```python
from build123d import *

# Parameters (mm, degrees)
EXTRUDE_1_REACH          = 90.826
EXTRUDE_1_END_RADIUS     = 27
SKETCH_2_R               = 13
SKETCH_4_R               = 9
CUT_EXTRUDE_2_DEPTH      = 89.825671965
SKETCH_5_R               = 10
CUT_EXTRUDE_3_DEPTH      = 0.5
EXTRUDE_1_2_REACH        = 90.826
CUT_EXTRUDE_4_DEPTH      = 82.737384446
CUT_EXTRUDE_4_DEPTH_BACK = 82.737384446
SKETCH_6_W               = 70
SKETCH_6_H               = 5


with BuildPart() as part:
    # 草图1 → 旋转1 (revolve)
    with BuildSketch(Plane.XY, mode=Mode.PRIVATE) as revolve_1_sk:
        with BuildLine():
            Line((0, 53), (25, 53))
            ThreePointArc((25, 53), (28.535533906, 54.464466094), (30, 58))
            Line((30, 58), (30, 59))
            Line((30, 59), (40, 59))
            Line((40, 59), (40, 53))
            Line((40, 53), (37, 53))
            Line((37, 53), (37, 51))
            Line((37, 51), (40, 51))
            Line((40, 51), (40, 48))
            Line((40, 48), (37, 48))
            Line((37, 48), (37, 46))
            Line((37, 46), (40, 46))
            Line((40, 46), (40, 44))
            Line((40, 44), (37, 44))
            Line((37, 44), (37, 41))
            Line((37, 41), (40, 41))
            Line((40, 41), (40, 0))
            Line((40, 0), (27, 0))
            Line((27, 0), (27, 41.5))
            ThreePointArc((27, 41.5), (25.535533906, 45.035533906), (22, 46.5))
            Line((22, 46.5), (0, 46.5))
            Line((0, 46.5), (0, 53))
        make_face()
    revolve(revolve_1_sk.sketch.rotate(Axis((0, -5, 0), (0, 1, 0)), 90), axis=Axis((0, -5, 0), (0, 1, 0)))

    # Extrude 1: up to this cylinder (the profile starts inside it)
    extrude_1_end = Plane(origin=(0, 25, 0), z_dir=(0, -1, 0)) * Cylinder(EXTRUDE_1_END_RADIUS, 236.652, mode=Mode.PRIVATE)
    # 草图2 → Extrude 1 (add, up to the surface)
    with BuildSketch(Plane.XY.offset(13), mode=Mode.PRIVATE) as extrude_1_sk1:
        with Locations(Location((0, 25, 0), (0, 0, 180))):
            Circle(SKETCH_2_R)
    extrude_1_tool1 = extrude(extrude_1_sk1.sketch, amount=EXTRUDE_1_REACH, mode=Mode.PRIVATE) & extrude_1_end
    extrude_1 = extrude_1_tool1.solids().sort_by_distance((0, 25, 13))[0]
    add(extrude_1)

    # 草图4 → 切除-拉伸2 (cut, through all)
    with BuildSketch(Plane.XY.offset(13)):
        with Locations(Location((0, 25, 0), (0, 0, 270))):
            Circle(SKETCH_4_R)
    cut_extrude_2 = extrude(amount=CUT_EXTRUDE_2_DEPTH, mode=Mode.SUBTRACT)

    # 草图5 → 切除-拉伸3 (cut)
    with BuildSketch(Plane.XY.offset(38)):
        with Locations((0, 25)):
            Circle(SKETCH_5_R)
    cut_extrude_3 = extrude(amount=CUT_EXTRUDE_3_DEPTH, mode=Mode.SUBTRACT)

    # 草图7 → Extrude 1 2 (add, up to next)
    with BuildSketch(Plane(origin=(0, 0, 13), x_dir=(-1, 0, 0), z_dir=(0, 0, -1)), mode=Mode.PRIVATE) as extrude_1_2_sk1:
        with BuildLine():
            Line((-13, 25), (-13, 46.5))
            Line((-13, 46.5), (13, 46.5))
            Line((13, 46.5), (13, 25))
            ThreePointArc((13, 25), (0, 38), (-13, 25))
        make_face()
    extrude_1_2_tool1 = extrude(extrude_1_2_sk1.sketch, amount=-EXTRUDE_1_2_REACH, mode=Mode.PRIVATE) - part.part
    extrude_1_2 = extrude_1_2_tool1.solids().sort_by_distance((0, 40.482231, 13))[0]
    add(extrude_1_2)

    # 镜向1: Extrude 1, 切除-拉伸2, 切除-拉伸3, Extrude 1 2 across plane
    add(extrude_1.mirror(Plane.XY))
    add(cut_extrude_2.mirror(Plane.XY), mode=Mode.SUBTRACT)
    add(cut_extrude_3.mirror(Plane.XY), mode=Mode.SUBTRACT)
    add(extrude_1_2.mirror(Plane.XY))

    # 草图6 → 切除-拉伸4 (cut, two sides: drawn at the far end of the back side and taken through both)
    with BuildSketch(Plane.XY.offset(-CUT_EXTRUDE_4_DEPTH_BACK)):
        with Locations((0, 2.5)):
            Rectangle(SKETCH_6_W, SKETCH_6_H)
    extrude(amount=CUT_EXTRUDE_4_DEPTH + CUT_EXTRUDE_4_DEPTH_BACK, mode=Mode.SUBTRACT)


solid = part.part
```
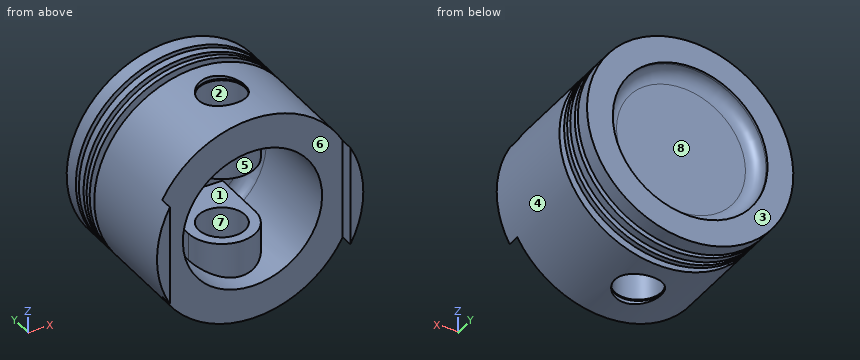
CAD build for the part. Positions are in the model's coordinates, mm. Face numbers are marked on the shaded views. A direction names the side the tool comes from. Round coordinates to 2 decimals unless told otherwise and drop trailing zeros. Order: outer loops, then holes, each group sorted by start corner. A loop starts at its lowest first (then second) coordinate and runs counter-clockwise, first axis right, second up.
Item 1: Mould opens along X. For the marked faces 1, 2, 3 and 4 say: pulls with the +X half, pulls with the -X half, needs draft (parallel to the pull), parting line crosses it, or undercut.
Item 2: Tool access for the marked faces 5, 6, 7 and 8: list every direction of +Z, -Z, +X, -X, +Y, -Y with a clear straight run to the whole face (end or side of a thin tool).
Item 3: Saw through at C-C on y = 8.5. Write the cut outline in (x, z), then the cut area to 3 significant figures.
Item 4: Saw through at B-B on x = 0. State how many separate pieces and enclosed holes the cut face has, then the cut area to 3 significant figures.
Item 5: Probe line 1 along Y through (x, z) = (0, 39); line 2 along Y through (x, z) = (-19, 32.5); line 3 along X through (y, z) = (25, 18). List the from-to ranges inside material, lowest first.
Item 6: Pin check, flat tips, straight feed: pin 1 (8.5 mm diameter, centred on y = 32, z = -17.5, fed in from +X); pin 2 (11 mm diameter, centred on x = 0, y = 25, fed in from -Z); pin 3 (4 mm diameter, centred on x = -6, y = 30, fed in from -Z); pin 4 (21 mm diameter, centred on x = 1, y = 26, fed in from -Z). Stop position of each tip, or through.
Reported:
1. face 1: undercut
1. face 2: undercut
1. face 3: needs draft
1. face 4: parting line crosses it
2. face 5: -Y
2. face 6: +Z, -Z, -Y
2. face 7: +Z, -Z
2. face 8: +Y
3. outline: circle Ø80 at (0, 0); hole circle Ø54 at (0, 0)
3. area: 2,740 mm2
4. separate pieces: 3
4. enclosed holes: 0
4. area: 1,680 mm2
5. line 1: y = 5 to 16, 34 to 41, 44 to 46, 48 to 51, 53 to 59
5. line 2: y = 5 to 41, 44 to 46, 48 to 51, 53 to 59
5. line 3: x = -35.72 to -20.12, -13 to -9, 9 to 13, 20.12 to 35.72
6. pin 1: stops at x = 37.74
6. pin 2: passes through
6. pin 3: stops at z = -39.59
6. pin 4: stops at z = -40
